from build123d import *

# Parameters (mm, degrees)
F0_W            = 20
F0_H            = 20
F1_DEPTH        = 50
F5_R            = 3
F6_SIZE         = 2
F7_R            = 3.5
F8_DEPTH        = 40
F10_D           = 4.4
F10_DEPTH       = 10
F10_CBORE_D     = 8.25
F10_CBORE_DEPTH = 4
F10_TIP         = 1.3218933619
F11_R           = 2
F12_DEPTH       = 27


with BuildPart() as f1:
    # F0 (on Top) → F1 (new body)
    with BuildSketch(Plane.XY):
        with Locations((0.1188712195, -1.538979894)):
            Rectangle(F0_W, F0_H)
    extrude(amount=F1_DEPTH)

    # F4: sweep along a path in F3
    with BuildLine(Plane.YZ) as f4_path:
        Line((-11.538979894, 0), (-16.538979894, 0))
        ThreePointArc((-16.538979894, 0), (-17.9531934564, -0.5857864376), (-18.538979894, -2))
        Line((-18.538979894, -2), (-18.538979894, -15))
    # F2 (on face) → F4 (sweep)
    with BuildSketch(Plane.XZ.offset(11.538979894)):
        with BuildLine():
            Line((-4, 7), (-4, 4))
            ThreePointArc((-4, 4), (-2.8284271247, 1.1715728753), (0, 0))
            ThreePointArc((0, 0), (2.8284271247, 1.1715728753), (4, 4))
            Line((4, 4), (4, 7))
            ThreePointArc((4, 7), (0, 11), (-4, 7))
        make_face()
    sweep(path=f4_path.line)

    # F5
    f5_edges = [f1.edges().sort_by_distance(p)[0] for p in [
        (-4, -24.03898, -15),
        (0, -18.53898, -15),
        (4, -24.03898, -15),
        (0, -29.53898, -15),
    ]]
    fillet(f5_edges, radius=F5_R)

    # F6
    f6_edges = [f1.edges().sort_by_distance(p)[0] for p in [
        (10.118871, -11.53898, 25),
        (10.118871, 8.46102, 25),
        (-9.881129, -11.53898, 25),
        (-9.881129, -1.53898, 0),
        (10.118871, -1.53898, 0),
        (0.118871, 8.46102, 0),
        (-9.881129, 8.46102, 25),
        (10.118871, -1.53898, 50),
        (0.118871, 8.46102, 50),
        (-9.881129, -1.53898, 50),
        (0.118871, -11.53898, 50),
    ]]
    chamfer(f6_edges, length=F6_SIZE)

    # F7 (on face) → F8 (cut)
    with BuildSketch(Plane.XY.offset(50)):
        with Locations((0, -0.538979894)):
            Circle(F7_R)
    extrude(amount=-F8_DEPTH, mode=Mode.SUBTRACT)

    # F10
    with Locations(Plane(origin=(0, 8.461020106, 0), x_dir=(-1, 0, 0), z_dir=(0, 1, 0))):
        with Locations((0, 40), (0, 30), (0, 20)):
            CounterBoreHole(F10_D / 2, F10_CBORE_D / 2, F10_CBORE_DEPTH, depth=F10_DEPTH)
            with Locations((0, 0, -(F10_DEPTH + F10_TIP / 2))):  # 118° drill point
                Cone(0, F10_D / 2, F10_TIP, mode=Mode.SUBTRACT)

    # F11 (on face) → F12 (cut)
    with BuildSketch(Plane(origin=(0, 8.461020106, 0), x_dir=(-1, 0, 0), z_dir=(0, 1, 0))):
        with Locations((0, 5)):
            Circle(F11_R)
    extrude(amount=-F12_DEPTH, mode=Mode.SUBTRACT)


solid = f1.part
The listing builds one solid part. Answer for the finished solid, in the listing's coordinates (mm). A direction names the side the tool comes from. Coordinates: 2 decimals unless noted, no trailing zeros. Order: outer loops, then holes, each group sorted by start corner. A loop starts at its lowest first (then second) coordinate and runs counter-clockwise, first axis right, second up. Notation, with made-up numbers: (78.25, 44) -> (104.25, 44) arc R20 ccw to (104.25, 68) -> close; hole circle Ø7 at (22, -15). An arc over 180 degrees is marked (long way). Answer in a Markdown table with one row per item. Add a question column.
Item 1: Which of the six approach directions +Z, -Z, +X, -X, +Y, -Y give full straight-line access (tool end or side, diameter ignored) to faces 1 (the face through (0, -24, -15)), 2 (the face through (-2, 4.461, 18)), 3 (the face through (4, -23, 0))?
Item 2: Find section A-A (z = 30). Write down the section's boundary in (x, y) (3 decimals), then the cut area to 3 significant figures.
Item 3: Find section C-C (y = -2.5). Write down the section's boundary in (x, z).
Item 4: Determine the mould class of faces 4 (the face through (-3.14, -24.02, -14.1)), 5 (the face through (-8.49, 7.22, 1.37)), 6 (the face through (-0.759, -3.956, 30.28)) for opening direction Y: +Y half, -Y half, draft (parallel to the pull), parting line (faces both ways), or undercut.
Item 5: Find the intervals of material crossed by L1, parallel to Z at x = 0, y = 5.3 (3 decimals); L2, parallel to Z at x = 0, y = -12; L3, parallel to X at y = 2.8, z = 40, in increasing order. Write a range as from..to.
Item 6: Find section B-B (x = -7). Write down the section's boundary in (y, z), then the cut area to 3 significant figures.
Item 7: Find section D-D (z = 46). Write down the section's boundary in (x, y), then the cut area to 3 significant figures.
Item 8: Each of these flat-tipped pins is pushed along its axis until it touches: P1, Ø3.5, axis at x = 0, z = 40, coming from the -Y side; P2, Ø1, axis at x = -4.5, y = 4.5, coming from the -Z side; P3, Ø5.5, axis at x = 0, y = -0.54, coming from the +Z side. Where does it stop, or does it pass through?
Result set:
| question | item | result |
|---|---|---|
| 1 | face 1 | -Z, +X, -X, +Y, -Y |
| 1 | face 2 | +Y |
| 1 | face 3 | +Z, -Z, +X, -Y |
| 2 | outline | (-9.881, -9.539) -> (-7.881, -11.539) -> (8.119, -11.539) -> (10.119, -9.539) -> (10.119, 6.461) -> (8.119, 8.461) -> (4.125, 8.461) -> (4.125, 4.461) -> (2.2, 4.461) -> (2.2, 2.183) arc R3.5 cw (long way) to (-2.2, 2.183) -> (-2.2, 4.461) -> (-4.125, 4.461) -> (-4.125, 8.461) -> (-7.881, 8.461) -> (-9.881, 6.461) -> close |
| 2 | area | 313 mm² |
| 3 | outline | (-9.88, 2) -> (-7.88, 0) -> (8.12, 0) -> (10.12, 2) -> (10.12, 48) -> (8.12, 50) -> (2.9, 50) -> (2.9, 10) -> (-2.9, 10) -> (-2.9, 50) -> (-7.88, 50) -> (-9.88, 48) -> close; hole circle Ø4 at (0, 5) |
| 4 | face 4 | draft |
| 4 | face 5 | +Y half |
| 4 | face 6 | undercut |
| 5 | L1 | z = 0..3, 7..15.875, 24.125..25.875, 34.125..35.875, 44.125..50 |
| 5 | L2 | z = 0..3, 7..11 |
| 5 | L3 | x = -9.88..-2.2, 2.2..10.12 |
| 6 | outline | (-11.54, 0) -> (6.46, 0) -> (8.46, 2) -> (8.46, 48) -> (6.46, 50) -> (-9.54, 50) -> (-11.54, 48) -> close |
| 6 | area | 994 mm² |
| 7 | outline | (-9.88, -9.54) -> (-7.88, -11.54) -> (8.12, -11.54) -> (10.12, -9.54) -> (10.12, 6.46) -> (8.12, 8.46) -> (-7.88, 8.46) -> (-9.88, 6.46) -> close; hole circle Ø7 at (0, -0.54) |
| 7 | area | 354 mm² |
| 8 | P1 | stops at y = -11.54 |
| 8 | P2 | stops at z = 0 |
| 8 | P3 | stops at z = 10 |
